```python
from build123d import *

# Parameters (mm, degrees)
F0_W     = 63
F0_H     = 90
F1_DEPTH = 1.6
F2_R     = 1.1303
F3_DEPTH = 25


with BuildPart() as f1:
    # F0 (on Top) → F1 (new body)
    with BuildSketch(Plane.XY):
        Rectangle(F0_W, F0_H)
    extrude(amount=F1_DEPTH)

    # F2 (on face) → F3 (cut)
    with BuildSketch(Plane.XY.offset(1.6)):
        with Locations((-28, 41.5)):
            Circle(F2_R)
        with Locations((0, 41.5)):
            Circle(F2_R)
        with Locations((28, 41.5)):
            Circle(F2_R)
        with Locations((28, 13.833333)):
            Circle(F2_R)
        with Locations((28, -13.833333)):
            Circle(F2_R)
        with Locations((0, -41.5)):
            Circle(F2_R)
        with Locations((-28, -41.5)):
            Circle(F2_R)
        with Locations((-28, -13.833333)):
            Circle(F2_R)
        with Locations((-28, 13.833333)):
            Circle(F2_R)
        with Locations((28, -41.5)):
            Circle(F2_R)
    extrude(amount=-F3_DEPTH, mode=Mode.SUBTRACT)


solid = f1.part
```
Work out the finished part from the listing and answer in its coordinate system (mm). Give positions to 0.01 mm unless a question says otherwise; leave off trailing zeros. Write each loop counter-clockwise with the first axis right and the second up, starting at its lowest first coordinate (ties: lowest second). Pieces come first, ordered by that corner, then holes. Notation, with made-up numbers: (73.5, 58.25) -> (105.5, 58.25) arc R23 cw to (105.5, 83.25) -> close; hole circle Ø11 at (-24, -12). An arc over 180 degrees is marked (long way). Write each question's results on one line, items separated by ' | '.
1. Find section C-C on x = 28. Determine the outline of the cut face in (y, z), and give its area (3 significant figures).
Data:
outline: (-45, 0) -> (-42.63, 0) -> (-42.63, 1.6) -> (-45, 1.6) -> close; (-40.37, 0) -> (-14.96, 0) -> (-14.96, 1.6) -> (-40.37, 1.6) -> close; (-12.7, 0) -> (12.7, 0) -> (12.7, 1.6) -> (-12.7, 1.6) -> close; (14.96, 0) -> (40.37, 0) -> (40.37, 1.6) -> (14.96, 1.6) -> close; (42.63, 0) -> (45, 0) -> (45, 1.6) -> (42.63, 1.6) -> close | area: 130 mm^2
2. Find section A-A on x = 0. Determine the outline of the cut face in (y, z).
Data:
outline: (-45, 0) -> (-42.63, 0) -> (-42.63, 1.6) -> (-45, 1.6) -> close; (-40.37, 0) -> (40.37, 0) -> (40.37, 1.6) -> (-40.37, 1.6) -> close; (42.63, 0) -> (45, 0) -> (45, 1.6) -> (42.63, 1.6) -> close
3. This flat-tipped pin is pushed along its axis until it touches: pin 1 Ø2.5 at (x, y) = (28, -41.5) entering from +Z. Where does it stop, or does it pass through?
Data:
pin 1: z = 1.6
4. Straight lines are drawn through the part: L1, parallel to Y at x = -28, z = 0.6; L2, parallel to Y at x = 0, z = 0.75; L3, parallel to Y at x = 1, z = 1. For each, find the intervals that lie inside material, in ascending order.
Data:
L1: -45 to -42.63, -40.37 to -14.96, -12.7 to 12.7, 14.96 to 40.37, 42.63 to 45 | L2: -45 to -42.63, -40.37 to 40.37, 42.63 to 45 | L3: -45 to -42.03, -40.97 to 40.97, 42.03 to 45
5. Find section B-B on y = -41.5. Determine the outline of the cut face in (x, z), and give its area (3 significant figures).
Data:
outline: (-31.5, 0) -> (-29.13, 0) -> (-29.13, 1.6) -> (-31.5, 1.6) -> close; (-26.87, 0) -> (-1.13, 0) -> (-1.13, 1.6) -> (-26.87, 1.6) -> close; (1.13, 0) -> (26.87, 0) -> (26.87, 1.6) -> (1.13, 1.6) -> close; (29.13, 0) -> (31.5, 0) -> (31.5, 1.6) -> (29.13, 1.6) -> close | area: 89.9 mm^2
6. Determine the mould class of faces 1 (the flat face through (0, 1, 0)), 2 (the cylindrical face through (26.87, 13.88, 0.81)) for opening direction X: +X half, -X half, draft (parallel to the pull), parting line (faces both ways), or undercut.
Data:
face 1: draft | face 2: undercut
